Build history of the part. All positions in model axes, mm. A direction names the side the tool comes from. Give positions to 0.01 mm unless a question says otherwise; leave off trailing zeros. Order: outer loops, then holes, each group sorted by start corner. A loop starts at its lowest first (then second) coordinate and runs counter-clockwise, first axis right, second up. Notation, with made-up numbers: (47, 59.25) - (96, 59.25) arc R26 cw to (96, 88.25) - close; hole circle Ø3 at (52.25, -28.5). An arc over 180 degrees is marked (long way). Answer in a Markdown table with one row per item.
```python
from build123d import *

# Parameters (mm, degrees)
SKETCH1_W               = 1.27
SKETCH1_H               = 6.35
SKETCH1_H_2             = 3.175
BOSS_EXTRUDE1_DEPTH     = 27.94
CUT_EXTRUDE1_DEPTH      = 62.500004065
CUT_EXTRUDE1_DEPTH_BACK = 62.500004065
SKETCH2_R               = 1.5
SKETCH2_R_2             = 1.554918768
SKETCH2_R_3             = 1.519223358
SKETCH2_3_R             = 1.8175
SKETCH2_3_R_2           = 1.5
SKETCH2_3_R_3           = 1.872418768
SKETCH2_3_R_4           = 1.554918768
SKETCH2_3_R_5           = 1.836723358
SKETCH2_3_R_6           = 1.519223358
CUT_EXTRUDE2_DEPTH      = 17.78
BOSS_EXTRUDE2_START     = -0.6858
SKETCH1_2_W             = 1.27
SKETCH1_2_H             = 6.35
SKETCH1_2_H_2           = 3.175
BOSS_EXTRUDE2_DEPTH     = 0.6858


with BuildPart() as part:
    # Sketch1 → Boss-Extrude1 (new body)
    with BuildSketch(Plane(origin=(0, 0, 0), x_dir=(1, 0, 0), z_dir=(0, 1, 0))):
        with BuildLine():
            ThreePointArc((69.528895746, -31.115), (94.825388136, -2.928413856), (75.136623327, 29.425082184))
            ThreePointArc((75.136623327, 29.425082184), (72.134335795, 30.470176889), (69.042587949, 31.209804239))
            Line((69.042587949, 31.209804239), (70.208960434, 37.451765087))
            ThreePointArc((70.208960434, 37.451765087), (101.148320659, -3.514096627), (63.210725521, -38.1))
            Line((63.210725521, -38.1), (63.210725521, -31.75))
            ThreePointArc((63.210725521, -31.75), (66.385725521, -31.590851128), (69.528895746, -31.115))
        make_face()
        Polygon((67.794195779, 31.443078736), (67.211009536, 28.322098312), (68.459401706, 28.088823815), (69.042587949, 31.209804239), align=None)
        Polygon((67.794195779, 31.443078736), (68.960568265, 37.685039584), (70.208960434, 37.451765087), (69.042587949, 31.209804239), align=None)
        with Locations((62.575725521, -34.925)):
            Rectangle(SKETCH1_W, SKETCH1_H)
        with Locations((62.575725521, -30.1625)):
            Rectangle(SKETCH1_W, SKETCH1_H_2)
    extrude(amount=BOSS_EXTRUDE1_DEPTH)

    # Sketch2 → Cut-Extrude1 (cut, two sides: drawn at the far end of the back side and taken through both)
    with BuildSketch(Plane.ZY.offset(-61.940725521).offset(-CUT_EXTRUDE1_DEPTH_BACK)):
        with Locations((34.877492102, 15.559033415)):
            Circle(SKETCH2_R)
        with Locations((35.191543991, 24.633934205)):
            Circle(SKETCH2_R_2)
        with Locations((-35.170796856, 24.633934205)):
            Circle(SKETCH2_R_3)
        with Locations((-35.170796856, 15.364007333)):
            Circle(SKETCH2_R)
    extrude(amount=CUT_EXTRUDE1_DEPTH + CUT_EXTRUDE1_DEPTH_BACK, mode=Mode.SUBTRACT)

    # Sketch2_3 → Cut-Extrude2 (cut)
    # profile 1 of 4: a face of its own
    with BuildSketch(Plane.ZY.offset(-61.940725521)):
        with Locations((34.877492102, 15.559033415)):
            Circle(SKETCH2_3_R)
        with Locations((34.877492102, 15.559033415)):
            Circle(SKETCH2_3_R_2, mode=Mode.SUBTRACT)
    # profile 2 of 4: a face of its own
    with BuildSketch(Plane.ZY.offset(-61.940725521)):
        with Locations((35.191543991, 24.633934205)):
            Circle(SKETCH2_3_R_3)
        with Locations((35.191543991, 24.633934205)):
            Circle(SKETCH2_3_R_4, mode=Mode.SUBTRACT)
    # profile 3 of 4: a face of its own
    with BuildSketch(Plane.ZY.offset(-61.940725521)):
        with Locations((-35.170796856, 24.633934205)):
            Circle(SKETCH2_3_R_5)
        with Locations((-35.170796856, 24.633934205)):
            Circle(SKETCH2_3_R_6, mode=Mode.SUBTRACT)
    # profile 4 of 4: a face of its own
    with BuildSketch(Plane.ZY.offset(-61.940725521)):
        with Locations((-35.170796856, 15.364007333)):
            Circle(SKETCH2_3_R)
        with Locations((-35.170796856, 15.364007333)):
            Circle(SKETCH2_3_R_2, mode=Mode.SUBTRACT)
    extrude(amount=-CUT_EXTRUDE2_DEPTH, mode=Mode.SUBTRACT)

    # Sketch1_2 → Boss-Extrude2 (add)
    with BuildSketch(Plane(origin=(0, 0, 0), x_dir=(1, 0, 0), z_dir=(0, 1, 0)).offset(BOSS_EXTRUDE2_START)):
        with BuildLine():
            ThreePointArc((69.528895746, -31.115), (94.825388136, -2.928413856), (75.136623327, 29.425082184))
            ThreePointArc((75.136623327, 29.425082184), (72.134335795, 30.470176889), (69.042587949, 31.209804239))
            Line((69.042587949, 31.209804239), (70.208960434, 37.451765087))
            ThreePointArc((70.208960434, 37.451765087), (101.148320659, -3.514096627), (63.210725521, -38.1))
            Line((63.210725521, -38.1), (63.210725521, -31.75))
            ThreePointArc((63.210725521, -31.75), (66.385725521, -31.590851128), (69.528895746, -31.115))
        make_face()
        Polygon((67.794195779, 31.443078736), (68.960568265, 37.685039584), (70.208960434, 37.451765087), (69.042587949, 31.209804239), align=None)
        Polygon((67.794195779, 31.443078736), (67.211009536, 28.322098312), (68.459401706, 28.088823815), (69.042587949, 31.209804239), align=None)
        with Locations((62.575725521, -34.925)):
            Rectangle(SKETCH1_2_W, SKETCH1_2_H)
        with Locations((62.575725521, -30.1625)):
            Rectangle(SKETCH1_2_W, SKETCH1_2_H_2)
    extrude(amount=BOSS_EXTRUDE2_DEPTH)


solid = part.part
```
1. Probe line 1 (Z direction, x = 67, y = 16.25); line 2 (X direction, y = 9, z = 1); line 3 (Z direction, x = 85, y = 9.25). List the from-to ranges inside material, lowest first.
Check result:
| item | result |
|---|---|
| line 1 | z = 31.52 to 33.2, 36.56 to 37.91 |
| line 2 | x = 94.94 to 101.3 |
| line 3 | z = -31.25 to -23.09, 23.09 to 31.25 |
2. Which spindle directions (+Z, -Z, +X, -X, +Y, -Y) get a long thin tool onto all of the face, cutting with end or side? Do faces 1 (the face through (63.211, 13, 30)), 2 (the face through (80.458, 15.584, 33.378)), 3 (the face through (68.747, 13.427, -29.627)), 4 (the face through (101.213, 13.427, 2.728)), 5 (the face through (72.569, 15.91, -33.437)). Say none if no direction does.
Check result:
| item | result |
|---|---|
| face 1 | -Z, +Y, -Y |
| face 2 | +Z, +X, -X |
| face 3 | +Y, -Y |
| face 4 | +X, +Y, -Y |
| face 5 | -X |
3. Two-plate mould, pull along Y, no slides. Class faces 6 (the face through (95, -0.686, 3)), 7 (the face through (68.1, 13.43, -33.07)), 8 (the face through (80.269, 24.655, 33.637)): +Y half, -Y half, draft (parallel to the pull), parting line (faces both ways), or undercut.
Check result:
| item | result |
|---|---|
| face 6 | -Y half |
| face 7 | draft |
| face 8 | undercut |
4. Cut at A-A on x = 86. Write the cut outline in (y, z), and give its area (3 significant figures).
Check result:
| item | result |
|---|---|
| outline | (-0.69, -30.53) - (27.94, -30.53) - (27.94, -22.11) - (-0.69, -22.11) - close; (-0.69, 22.11) - (27.94, 22.11) - (27.94, 30.53) - (-0.69, 30.53) - close |
| area | 482 mm² |
5. Cut at B-B on y = 11.5. Write the cut outline in (x, z) (3 decimals).
Check result:
| item | result |
|---|---|
| outline | (61.941, 28.575) - (63.211, 28.575) - (63.211, 31.75) arc R31.75 cw to (69.043, -31.21) - (68.459, -28.089) - (67.211, -28.322) - (68.961, -37.685) - (70.209, -37.452) arc R38.1 ccw to (63.211, 38.1) - (61.941, 38.1) - close |
6. Drop flat-ended pins along their axis: P1, Ø4.5, axis at y = 24.63, z = 35.19, coming from the +X side; P2, Ø1.4, axis at x = 62.5, y = 13.5, coming from the -Z side (3 decimals); P3, Ø1, axis at x = 70, y = 17, coming from the -Z side; P4, Ø10, axis at x = 80, z = -16, coming from the +Y side (1 decimal). Give the stop position or say it passes through.
Check result:
| item | result |
|---|---|
| P1 | stops at x = 82.36 |
| P2 | stops at z = 28.575 |
| P3 | stops at z = -37.58 |
| P4 | passes through |
7. Cut at D-D on z = 25. Write the cut outline in (x, y).
Check result:
| item | result |
|---|---|
| outline | (82.78, -0.69) - (91.96, -0.69) - (91.96, 27.94) - (82.78, 27.94) - close |
8. Cut at C-C on x = 91. Write the cut outline in (y, z).
Check result:
| item | result |
|---|---|
| outline | (-0.69, -26.06) - (27.94, -26.06) - (27.94, -15.36) - (-0.69, -15.36) - close; (-0.69, 15.36) - (27.94, 15.36) - (27.94, 26.06) - (-0.69, 26.06) - close |
